from build123d import *

# Parameters (mm, degrees)
ESQUISSE1_R             = 26
BOSS_EXTRU_1_DEPTH      = 40
ENL_V_MAT_EXTRU_1_REACH = 184.502
ESQUISSE3_R             = 3.3
ENL_V_MAT_EXTRU_2_DEPTH = 179.283669838


with BuildPart() as part:
    # Esquisse1 → Boss.-Extru.1 (new body)
    with BuildSketch(Plane.XY):
        Polygon((-165.774144338, -1.493499921), (-80.774144338, -1.493499921), (-80.774144338, 50.506500079), (-96.774144338, 50.506500079), (-109.274144338, 65.006500079), (-137.274144338, 65.006500079), (-149.774144338, 50.506500079), (-165.774144338, 50.506500079), align=None)
        with Locations((-123.274144338, 31.756500079)):
            Circle(ESQUISSE1_R, mode=Mode.SUBTRACT)
    extrude(amount=BOSS_EXTRU_1_DEPTH)

    # Esquisse2 → Enlèv. mat.-Extru.1 (cut, up to next)
    with BuildSketch(Plane.XY.offset(40), mode=Mode.PRIVATE) as enl_v_mat_extru_1_sk1:
        with BuildLine():
            Line((-97.293382224, 32.756500079), (-80.774144338, 32.756500079))
            Line((-80.774144338, 32.756500079), (-80.774144338, 30.756500079))
            Line((-80.774144338, 30.756500079), (-97.293382224, 30.756500079))
            ThreePointArc((-97.293382224, 30.756500079), (-97.274144338, 31.756500079), (-97.293382224, 32.756500079))
        make_face()
    enl_v_mat_extru_1_tool1 = extrude(enl_v_mat_extru_1_sk1.sketch, amount=-ENL_V_MAT_EXTRU_1_REACH, mode=Mode.PRIVATE) & part.part
    add(enl_v_mat_extru_1_tool1.solids().sort_by_distance((-89.027351, 31.7565, 40))[0], mode=Mode.SUBTRACT)

    # Esquisse3 → Enlèv. mat.-Extru.2 (cut, through all)
    with BuildSketch(Plane(origin=(0, 50.506500079, 0), x_dir=(1, 0, 0), z_dir=(0, 1, 0))):
        with Locations(Location((-158.274144338, -10, 0), (0, 0, 270))):
            Circle(ESQUISSE3_R)
        with Locations(Location((-158.274144338, -30, 0), (0, 0, 270))):
            Circle(ESQUISSE3_R)
        with Locations(Location((-88.274144338, -10, 0), (0, 0, 270))):
            Circle(ESQUISSE3_R)
        with Locations(Location((-88.274144338, -30, 0), (0, 0, 270))):
            Circle(ESQUISSE3_R)
    extrude(amount=-ENL_V_MAT_EXTRU_2_DEPTH, mode=Mode.SUBTRACT)


solid = part.part
Could you check a few things on this model? Use its own coordinates, in mm. A direction names the side the tool comes from. Give positions to 0.01 mm unless a question says otherwise; leave off trailing zeros. Loops run counter-clockwise (first coordinate to the right, second up) from the corner with the lowest first, then second, coordinate; pieces in that order, holes last. Notation, with made-up numbers: (23, -38) -> (78, -38) arc R23 ccw to (78, -25) -> close; hole circle Ø7 at (-16, 2.5). An arc over 180 degrees is marked (long way). Return JSON: item names as keys, results as strings.
Item 1: If we section it at A-A on z = 30: List the corners of the cut face in (x, y) for me, plus the area to 3 significant figures.
Geometry results:
{"outline": "(-165.77, -1.49) -> (-161.57, -1.49) -> (-161.57, 50.51) -> (-165.77, 50.51) -> close; (-154.97, -1.49) -> (-91.57, -1.49) -> (-91.57, 30.76) -> (-97.29, 30.76) arc R26 cw (long way) to (-97.29, 32.76) -> (-91.57, 32.76) -> (-91.57, 50.51) -> (-96.77, 50.51) -> (-109.27, 65.01) -> (-137.27, 65.01) -> (-149.77, 50.51) -> (-154.97, 50.51) -> close; (-84.97, -1.49) -> (-80.77, -1.49) -> (-80.77, 30.76) -> (-84.97, 30.76) -> close; (-84.97, 32.76) -> (-80.77, 32.76) -> (-80.77, 50.51) -> (-84.97, 50.51) -> close", "area": "2,180 mm²"}
Item 2: Which directions (+Z, -Z, +X, -X, +Y, -Y) give clear straight access to the entire face, cutting with the end or side of a thin tool? Please do faces 1 (the flat face through (-89, 30.757, 20)), 2 (the flat face through (-89, 50.507, 20)), 3 (the flat face through (-158, 50.507, 20)).
Geometry results:
{"face 1": "+Z, -Z, +X", "face 2": "+Z, -Z, +X, +Y", "face 3": "+Z, -Z, -X, +Y"}
Item 3: If we section it at B-B on y = 41: List the corners of the cut face in (x, z) for me, plus the area to 3 significant figures.
Geometry results:
{"outline": "(-165.77, 0) -> (-147.58, 0) -> (-147.58, 40) -> (-165.77, 40) -> close; (-98.97, 0) -> (-80.77, 0) -> (-80.77, 40) -> (-98.97, 40) -> close; hole circle Ø6.6 at (-158.27, 10); hole circle Ø6.6 at (-158.27, 30); hole circle Ø6.6 at (-88.27, 10); hole circle Ø6.6 at (-88.27, 30)", "area": "1,320 mm²"}
Item 4: If we section it at C-C on x = -112.5: List the corners of the cut face in (y, z) for me.
Geometry results:
{"outline": "(-1.49, 0) -> (8.09, 0) -> (8.09, 40) -> (-1.49, 40) -> close; (55.42, 0) -> (65.01, 0) -> (65.01, 40) -> (55.42, 40) -> close"}
Item 5: We'd pull the mould along Z, two halves only. Please class faces 4 (the cylindrical face through (-159.538, 24.871, 33.048)), 5 (the flat face through (-123, 65.007, 20)), 6 (the flat face through (-124, 3, 0)): +Z half, -Z half, draft (parallel to the pull), parting line (faces both ways), or undercut.
Geometry results:
{"face 4": "undercut", "face 5": "draft", "face 6": "-Z half"}
Item 6: I'm going to push flat-ended pins straight in: pin 1 (7.5 mm diameter, centred on x = -158.27, z = 30, fed in from +Y); pin 2 (2 mm diameter, centred on x = -93, y = 28.5, fed in from -Z). Where does each tip first touch, or does it pass through?
Geometry results:
{"pin 1": "stops at y = 50.51", "pin 2": "stops at z = 0"}
Item 7: I need wall thicknesses on L1, parallel to X at y = 11, z = 10; L2, parallel to X at y = 19.5, z = 32; L3, parallel to Y at x = -84.5, z = 11.5. Which ranges of each line are inside material? Lowest first, please. Write a range as from..to.
Geometry results:
{"L1": "x = -165.77..-161.57, -154.97..-138.93, -107.62..-91.57, -84.97..-80.77", "L2": "x = -165.77..-160.9, -155.65..-146.2, -100.34..-90.9, -85.65..-80.77", "L3": "y = -1.49..30.76, 32.76..50.51"}
Item 8: If we section it at D-D on y = 54: List the corners of the cut face in (x, z) for me.
Geometry results:
{"outline": "(-146.76, 0) -> (-136.74, 0) -> (-136.74, 40) -> (-146.76, 40) -> close; (-109.81, 0) -> (-99.79, 0) -> (-99.79, 40) -> (-109.81, 40) -> close"}
